Design review of the part built by this model. Coordinates are the model's own, in mm. A direction names the side the tool comes from. Give positions to 0.01 mm unless a question says otherwise; leave off trailing zeros. Write each loop counter-clockwise with the first axis right and the second up, starting at its lowest first coordinate (ties: lowest second). Pieces come first, ordered by that corner, then holes. Notation, with made-up numbers: (30.5, -37.75) - (83.5, -37.75) arc R22 cw to (83.5, -5.75) - close; hole circle Ø1 at (73.25, 0). An arc over 180 degrees is marked (long way). Write each question's results on one line, items separated by ' | '. Start each with the question number.
from build123d import *

# Parameters (mm, degrees)
EXTRUDE_1_DEPTH     = 5
CUT_EXTRUDE_1_DEPTH = 5
EXTRUDE_2_DEPTH     = 5
EXTRUDE_3_DEPTH     = 5
SKETCH_5_W          = 6
SKETCH_5_H          = 5
CUT_EXTRUDE_2_DEPTH = 1
SKETCH_6_W          = 5
SKETCH_6_H          = 6
CUT_EXTRUDE_3_DEPTH = 1


with BuildPart() as part:
    # 草图1 → 凸台-拉伸1 (new body)
    with BuildSketch(Plane.XY):
        Polygon((0, 0), (-20, 0), (0, 20), align=None)
    extrude(amount=EXTRUDE_1_DEPTH)

    # 草图2 → 切除-拉伸1 (cut)
    with BuildSketch(Plane.XY.offset(5)):
        Polygon((-8.585786438, 8.585786438), (-10, 10), (-20, 0), align=None)
        Polygon((-8.585786438, 8.585786438), (0, 20), (-10, 10), align=None)
    extrude(amount=-CUT_EXTRUDE_1_DEPTH, mode=Mode.SUBTRACT)

    # 草图3 → 凸台-拉伸2 (add)
    with BuildSketch(Plane.XZ):
        Polygon((-10, 0), (-13, 0), (-13, 5), (-7, 5), (-7, 0), align=None)
    extrude(amount=EXTRUDE_2_DEPTH)

    # 草图4 → 凸台-拉伸3 (add)
    with BuildSketch(Plane(origin=(0, 0, 0), x_dir=(0, 0, -1), z_dir=(1, 0, 0))):
        Polygon((0, 10), (0, 7), (-5, 7), (-5, 13), (0, 13), align=None)
    extrude(amount=EXTRUDE_3_DEPTH)

    # 草图5 → 切除-拉伸2 (cut)
    with BuildSketch(Plane.XZ.offset(5)):
        with Locations((-10, 2.5)):
            Rectangle(SKETCH_5_W, SKETCH_5_H)
    extrude(amount=-CUT_EXTRUDE_2_DEPTH, mode=Mode.SUBTRACT)

    # 草图6 → 切除-拉伸3 (cut)
    with BuildSketch(Plane(origin=(5, 0, 0), x_dir=(0, 0, -1), z_dir=(1, 0, 0))):
        with Locations((-2.5, 10)):
            Rectangle(SKETCH_6_W, SKETCH_6_H)
    extrude(amount=-CUT_EXTRUDE_3_DEPTH, mode=Mode.SUBTRACT)


solid = part.part
Q1. Insertion check: P1, Ø1.5, axis at x = -5.5, z = 2.5, coming from the +Y side; P2, Ø1.2, axis at x = 2, z = 1.5, coming from the -Y side; P3, Ø2, axis at y = -1.5, z = 3.5, coming from the -X side. Each pin has a flat end and moves straight along its axis. Give the tip position at first contact, or say it passes through.
Q2. Machinability: for faces 4 (the face through (2, 7, 2)), 5 (the face through (-13, -2, 2)), 6 (the face through (0, 17, 2)), 7 (the face through (-14.373, 4.233, 2.535)), which of the approach directions +Z, -Z, +X, -X, +Y, -Y give a long, thin tool a straight path to every point of the face, cutting with its end or side? Answer none if there is none.
Q3. Add section B-B on x = -1.25. State the section outline as (y, z) points, plus the area to 3 significant figures.
Q4. Add section C-C on y = 2.75. State the section outline as (x, z) points.
Q5. The part is to be moulded in two halves that separate along Z. For faces 1 (the face through (-5, 6, 0)), 2 (the face through (-5, 6, 5)), 3 (the face through (2, 13, 3)), say which applies: +Z half, -Z half, draft (parallel to the pull), parting line (faces both ways), or undercut.
Q6. Add section A-A on z = 1.6. State the section outline as (x, y) points.
Q7. For line 1 along Y through (x, z) = (3, 1.7); line 2 along X through (y, z) = (-0.75, 1.05); line 3 along X through (y, z) = (17, 3.5), list the stretches that pass through material, from the lowest coordinate up. Write a range as [from, to].
Result:
1) P1: stops at y = 13.69 | P2: stops at y = 7 | P3: stops at x = -13
2) face 4: +Z, -Z, +X, -Y | face 5: +Z, -Z, -X, -Y | face 6: +Z, -Z, +X, +Y | face 7: +Z, -Z, -X, +Y
3) outline: (0, 0) - (18.34, 0) - (18.34, 5) - (0, 5) - close | area: 91.7 mm²
4) outline: (-16.34, 0) - (0, 0) - (0, 5) - (-16.34, 5) - close
5) face 1: -Z half | face 2: +Z half | face 3: draft
6) outline: (-20, 0) - (-13, 0) - (-13, -4) - (-7, -4) - (-7, 0) - (0, 0) - (0, 7) - (4, 7) - (4, 13) - (0, 13) - (0, 20) - (-8.59, 8.59) - close
7) line 1: y = [7, 13] | line 2: x = [-13, -7] | line 3: x = [-2.26, 0]
